Input: part model. Units: mm. Frame: model coordinates. A direction names the side the tool comes from. Coordinates: 2 decimals unless noted, no trailing zeros. Order: outer loops, then holes, each group sorted by start corner. A loop starts at its lowest first (then second) coordinate and runs counter-clockwise, first axis right, second up. Notation, with made-up numbers: (75.5, 32) -> (110.5, 32) arc R35 cw to (110.5, 69) -> close; hole circle Ø11 at (-4.5, 25.5). An arc over 180 degrees is marked (long way). Write each question's results on one line, items separated by ' | '.
```python
from build123d import *

# Parameters (mm, degrees)
F1_DEPTH  = 2
F2_W      = 17
F2_H      = 24
F3_DEPTH  = 1
F4_W      = 12
F4_H      = 15
F5_DEPTH  = 2.5
F6_W      = 8
F6_H      = 6
F7_DEPTH  = 3
F8_W      = 2
F8_H      = 4.5
F9_DEPTH  = 2
F10_W     = 2
F10_H     = 1
F11_DEPTH = 1
F12_W     = 10.5
F12_H     = 4
F13_DEPTH = 1.5
F14_R     = 0.375
F15_DEPTH = 25


with BuildPart() as f1:
    # F0 (on Top) → F1 (new body)
    with BuildSketch(Plane.XY):
        Polygon((13, 17), (-13, 17), (-13, -11), (-10, -11), (-10, -17), (13, -17), align=None)
    extrude(amount=F1_DEPTH)

    # F2 (on face) → F3 (join)
    with BuildSketch(Plane.XY.offset(2)):
        with Locations((0, 5)):
            Rectangle(F2_W, F2_H)
    extrude(amount=F3_DEPTH)

    # F4 (on face) → F5 (join)
    with BuildSketch(Plane.XY.offset(3)):
        with Locations((0, 1.5)):
            Rectangle(F4_W, F4_H)
    extrude(amount=F5_DEPTH)

    # F6 (on face) → F7 (join)
    with BuildSketch(Plane(origin=(0, 0, 0), x_dir=(1, 0, 0), z_dir=(0, 0, -1))):
        with Locations((0, 14)):
            Rectangle(F6_W, F6_H)
    extrude(amount=F7_DEPTH)

    # F8 (on face) → F9 (join)
    with BuildSketch(Plane(origin=(0, 0, 0), x_dir=(1, 0, 0), z_dir=(0, 0, -1))):
        with Locations((-9, 13.75)):
            Rectangle(F8_W, F8_H)
    extrude(amount=F9_DEPTH)

    # F10 (on face) → F11 (join)
    with BuildSketch(Plane(origin=(-10, 0, 0), x_dir=(0, -1, 0), z_dir=(-1, 0, 0))):
        with Locations((13.75, -1)):
            Rectangle(F10_W, F10_H)
    extrude(amount=F11_DEPTH)

    # F12 (on face) → F13 (join)
    with BuildSketch(Plane(origin=(0, 0, 0), x_dir=(1, 0, 0), z_dir=(0, 0, -1))):
        with Locations((-0.75, 0.206931)):
            Rectangle(F12_W, F12_H)
    extrude(amount=F13_DEPTH)

    # F14 (on face) → F15 (cut)
    with BuildSketch(Plane(origin=(0, 0, 0), x_dir=(1, 0, 0), z_dir=(0, 0, -1))):
        with Locations((-11.5, -9)):
            Circle(F14_R)
        with Locations((-11.5, -6.5)):
            Circle(F14_R)
        with Locations((-11.5, -4)):
            Circle(F14_R)
        with Locations((-11.5, -1.5)):
            Circle(F14_R)
        with Locations((-11.5, 1)):
            Circle(F14_R)
        with Locations((-11.5, 3.5)):
            Circle(F14_R)
        with Locations((-11.5, 6)):
            Circle(F14_R)
        with Locations((-11.5, 8.5)):
            Circle(F14_R)
        with Locations((11.5, -9)):
            Circle(F14_R)
        with Locations((11.5, -6.5)):
            Circle(F14_R)
        with Locations((11.5, -4)):
            Circle(F14_R)
        with Locations((11.5, -1.5)):
            Circle(F14_R)
        with Locations((11.5, 1)):
            Circle(F14_R)
        with Locations((11.5, 3.5)):
            Circle(F14_R)
        with Locations((11.5, 6)):
            Circle(F14_R)
        with Locations((11.5, 8.5)):
            Circle(F14_R)
    extrude(amount=-F15_DEPTH, mode=Mode.SUBTRACT)


solid = f1.part
```
(1) Line query: line 1 along X through (y, z) = (9, 1.1) (3 decimals); line 2 along X through (y, z) = (5, 5.25); line 3 along Z through (x, y) = (3.25, 8.5). Output: solid intervals per line, ascending. Write a range as from..to.
Return value:
line 1: -13..-11.875, -11.125..11.125, 11.875..13 | line 2: -6..6 | line 3: 0..5.5
(2) Mould query, pull axis X, two halves, no side actions, for faces 6 (the face through (4.5, 0, -1)), 7 (the face through (-8, -14, -1)), 8 (the face through (0, -6, 4)). Classes: +X half, -X half, draft (parallel to the pull), parting line (faces both ways), or undercut.
Return value:
face 6: +X half | face 7: undercut | face 8: draft
(3) Pin query (flat end, axial travel): P1, Ø3, axis at y = -13, z = -1, coming from the -X side; P2, Ø1.5, axis at y = -10.5, z = -1, coming from the -X side; P3, Ø0.6, axis at x = -9, z = -1, coming from the +Y side. Return the tip coordinate at first contact, or that it passes through.
Return value:
P1: x = -11 | P2: x = -4 | P3: y = -11.5
(4) Cut plane B-B, the plane x = -0.5. Return loops of the section in (y, z).
Return value:
outline: (-17, -3) -> (-11, -3) -> (-11, 0) -> (-2.21, 0) -> (-2.21, -1.5) -> (1.79, -1.5) -> (1.79, 0) -> (17, 0) -> (17, 3) -> (9, 3) -> (9, 5.5) -> (-6, 5.5) -> (-6, 3) -> (-7, 3) -> (-7, 2) -> (-17, 2) -> close
(5) Cut plane C-C, the plane z = 1. Count the separate pieces of the cut face and the enclosed holes in it, plus the area to 3 significant figures.
Return value:
separate pieces: 1 | enclosed holes: 16 | area: 859 mm2
(6) Reachability of faces 1 (the face through (-1, 1.793, -1)), 2 (the face through (4, -14, -1)), 3 (the face through (-9, -11.5, -1)), 4 (the face through (-8.5, 4.8, 2.5)), 5 (the face through (-9, -16, -1)) from +Z, -Z, +X, -X, +Y, -Y: full face, straight path, thin tool, end or side. Return the list, or none.
Return value:
face 1: -Z, +X, -X, +Y | face 2: -Z, +X, -Y | face 3: -Z, -X, +Y | face 4: +Z, -X, +Y, -Y | face 5: -Z, -X, -Y
(7) Cut plane D-D, the plane y = 14.5. Return loops of the section in (x, z).
Return value:
outline: (-13, 0) -> (13, 0) -> (13, 2) -> (8.5, 2) -> (8.5, 3) -> (-8.5, 3) -> (-8.5, 2) -> (-13, 2) -> close
(8) Cut plane A-A, the plane y = 6.5. Return loops of the section in (x, z) (3 decimals).
Return value:
outline: (-13, 0) -> (-11.875, 0) -> (-11.875, 2) -> (-13, 2) -> close; (-11.125, 0) -> (11.125, 0) -> (11.125, 2) -> (8.5, 2) -> (8.5, 3) -> (6, 3) -> (6, 5.5) -> (-6, 5.5) -> (-6, 3) -> (-8.5, 3) -> (-8.5, 2) -> (-11.125, 2) -> close; (11.875, 0) -> (13, 0) -> (13, 2) -> (11.875, 2) -> close
